The figure shows three views and two pictorial views of one solid part (mm, origin at its lowest corner). Answer the questions. Round coordinates to 2 decimals unless told otherwise and drop trailing zeros. Order: outer loops, then holes, each group sorted by start corner. A loop starts at its lowest first (then second) coordinate and runs counter-clockwise, first axis right, second up. Notation, with made-up numbers: (-16.75, 75) - (16.25, 75) arc R28 ccw to (16.25, 99) - close; hole circle Ø3 at (66.5, -24.75). An arc over 180 degrees is marked (long way). Write item = value, one per line.
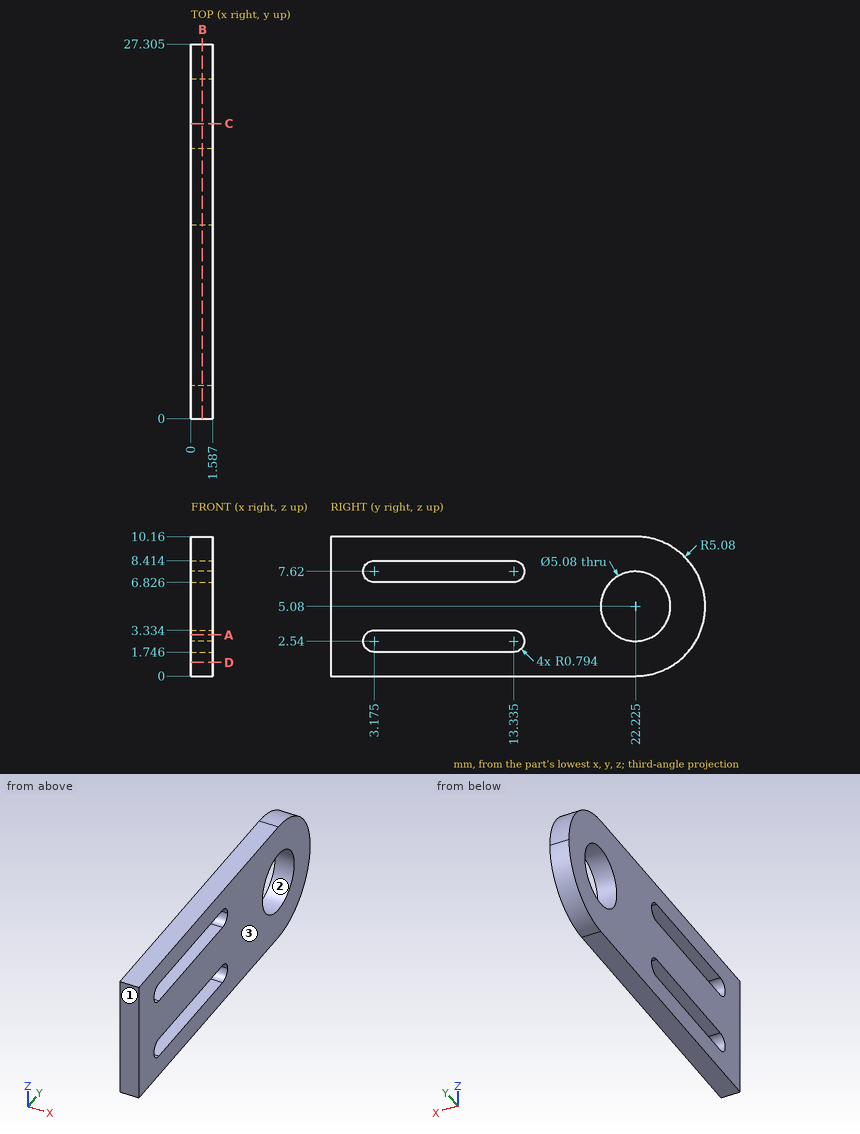
Q1. Determine the mould class of the marked faces 1, 2 and 3 for opening direction Y: released by +Y, released by -Y, zero draft, split by the parting line, or undercut.
Model answer:
face_1 = released by -Y
face_2 = undercut
face_3 = zero draft
Q2. Section D-D on z = 1 is taken. Determine the outline of the cut face in (x, y).
Model answer:
outline = (0, 0) - (1.59, 0) - (1.59, 25.25) - (0, 25.25) - close
Q3. Section C-C on y = 21.5 is taken. Determine the outline of the cut face in (x, z) (1 decimal).
Model answer:
outline = (0, 0) - (1.6, 0) - (1.6, 2.6) - (0, 2.6) - close; (0, 7.5) - (1.6, 7.5) - (1.6, 10.2) - (0, 10.2) - close
Q4. Find the intervals of material crossed by line 1 (Z direction, x = 0.5, y = 11.75); line 2 (Z direction, x = 0.7, y = 13.5) (1 decimal); line 3 (Y direction, x = 0.6, z = 3.25) (1 decimal), in increasing order. Write a range as from..to.
Model answer:
line_1 = 0..1.75, 3.33..6.83, 8.41..10.16
line_2 = 0..1.8, 3.3..6.8, 8.4..10.2
line_3 = 0..2.8, 13.7..20.5, 24..27
Q5. Section A-A on z = 3 is taken. Determine the outline of the cut face in (x, y).
Model answer:
outline = (0, 0) - (1.59, 0) - (1.59, 2.53) - (0, 2.53) - close; (0, 13.98) - (1.59, 13.98) - (1.59, 20.77) - (0, 20.77) - close; (0, 23.68) - (1.59, 23.68) - (1.59, 26.86) - (0, 26.86) - close
Q6. Section B-B on x = 0.85 is taken. Determine the outline of the cut face in (y, z) (1 decimal), then the cut area to 3 significant figures.
Model answer:
outline = (0, 0) - (22.2, 0) arc R5.1 ccw to (27.3, 5.1) arc R5.1 ccw to (22.2, 10.2) - (0, 10.2) - close; hole (3.2, 1.7) - (13.3, 1.7) arc R0.8 ccw to (13.3, 3.3) - (3.2, 3.3) arc R0.8 ccw to start; hole (3.2, 6.8) - (13.3, 6.8) arc R0.8 ccw to (13.3, 8.4) - (3.2, 8.4) arc R0.8 ccw to start; hole circle Ø5.1 at (22.2, 5.1)
area = 210 mm^2
